Source: CAD feature listing. Evaluate the final solid. Frame: model axes, mm. Face numbers are marked on the shaded views. Give positions to 0.01 mm unless a question says otherwise; leave off trailing zeros. Write each loop counter-clockwise with the first axis right and the second up, starting at its lowest first coordinate (ties: lowest second). Pieces come first, ordered by that corner, then holes.
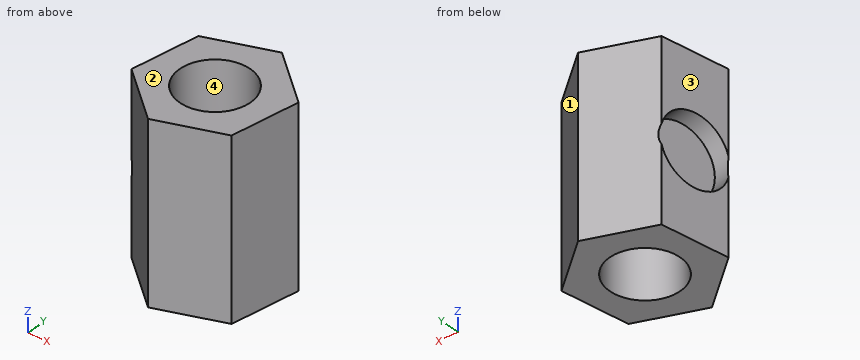
```python
from build123d import *

# Parameters (mm, degrees)
EXTRUDE_1_DEPTH     = 30
SKETCH_2_R          = 6
CUT_EXTRUDE_1_DEPTH = 34.854921873
SKETCH_4_R          = 6
CUT_EXTRUDE_2_DEPTH = 3


with BuildPart() as part:
    # Эскиз1 → Бобышка-Вытянуть1 (new body)
    with BuildSketch(Plane.XY):
        Polygon((8.992275581, -7.243777551), (10.769433169, 4.165650315), (1.777157588, 11.409427866), (-8.992275581, 7.243777551), (-10.769433169, -4.165650315), (-1.777157588, -11.409427866), align=None)
    extrude(amount=EXTRUDE_1_DEPTH)

    # Эскиз2 → Вырез-Вытянуть1 (cut, through all)
    with BuildSketch(Plane.XY.offset(30)):
        Circle(SKETCH_2_R)
    extrude(amount=-CUT_EXTRUDE_1_DEPTH, mode=Mode.SUBTRACT)

    # Эскиз4 → Вырез-Вытянуть2 (cut)
    with BuildSketch(Plane(origin=(-9.880854375, 1.539063618, 0), x_dir=(0, 0, 1), z_dir=(-0.9880854374988838, 0.15390636180041273, 0))):
        with Locations(Location((14.425169577, 0, 0), (0, 0, 270))):
            Circle(SKETCH_4_R)
    extrude(amount=-CUT_EXTRUDE_2_DEPTH, mode=Mode.SUBTRACT)


solid = part.part
```
1. Cut plane C-C, the plane z = 16.5. Return the cut outline in (x, y).
2. Contact query for flat-ended pins moving along their axis: P1, Ø2, axis at y = -9, z = 12, coming from the -X side; P2, Ø1, axis at y = 6, z = 20, coming from the -X side; P3, Ø12, axis at y = -8, z = 24.5, coming from the +X side. Output: stop coordinate, or through.
3. Cut plane D-D, the plane x = 3.25. Return the cut outline in (y, z), then the cut area to 3 significant figures.
4. Line query: L1, parallel to Y at x = -1, z = 22.75; L2, parallel to X at y = 3.5, z = 23; L3, parallel to Y at x = 0, z = 14. Output: solid intervals per line, ascending.
5. Cut plane A-A, the plane z = 3.25. Return the cut outline in (x, y), then the cut area to 3 significant figures.
6. Cut plane B-B, the plane x = 0. Return the cut outline in (y, z), then the cut area to 3 significant figures.
7. Mould query, pull axis X, two halves, no side actions, for the marked faces 1, 2, 3 and 4. Classes: +X half, -X half, draft (parallel to the pull), parting line (faces both ways), or undercut.
Response values:
1. outline: (-10.77, -4.17) - (-1.78, -11.41) - (8.99, -7.24) - (10.77, 4.17) - (1.78, 11.41) - (-8.99, 7.24) - (-9.01, 7.1) - (-6.05, 6.64) - (-7.78, -4.49) - (-10.75, -4.02) - close; hole circle Ø12 at (0, 0)
2. P1: stops at x = -6.01
2. P2: stops at x = -9.26
2. P3: stops at x = 9.81
3. outline: (-9.46, 0) - (-5.04, 0) - (-5.04, 30) - (-9.46, 30) - close; (5.04, 0) - (10.22, 0) - (10.22, 30) - (5.04, 30) - close
3. area: 288 mm2
4. L1: y = -11.11 to -5.92, 5.92 to 10.34
4. L2: x = -9.58 to -4.87, 4.87 to 10.67
4. L3: y = -10.72 to -6, 6 to 10.72
5. outline: (-10.77, -4.17) - (-1.78, -11.41) - (8.99, -7.24) - (10.77, 4.17) - (1.78, 11.41) - (-8.99, 7.24) - close; hole circle Ø12 at (0, 0)
5. area: 233 mm2
6. outline: (-10.72, 0) - (-6, 0) - (-6, 30) - (-10.72, 30) - close; (6, 0) - (10.72, 0) - (10.72, 30) - (6, 30) - close
6. area: 283 mm2
7. face 1: +X half
7. face 2: draft
7. face 3: -X half
7. face 4: undercut
